Work out the finished part from the listing and answer in its coordinate system (mm). A direction names the side the tool comes from. Coordinates: 2 decimals unless noted, no trailing zeros. Order: outer loops, then holes, each group sorted by start corner. A loop starts at its lowest first (then second) coordinate and runs counter-clockwise, first axis right, second up. Notation, with made-up numbers: M 64,31 L 74,31 A22 ccw 74,63 Z; hole C -20,74.5 d10. An arc over 180 degrees is marked long. Use a Markdown table: item, result.
from build123d import *

# Parameters (mm, degrees)
SKETCH_1_W          = 78
SKETCH_1_H          = 22.5
SKETCH_1_R          = 1
EXTRUDE_1_DEPTH     = 3
FILLET_1_R          = 5
SKETCH_2_R          = 1.5
SKETCH_2_W          = 20
SKETCH_2_H          = 6
EXTRUDE_2_DEPTH     = 3
SKETCH_4_R          = 1.5
CUT_EXTRUDE_1_DEPTH = 29.5
SKETCH_6_R          = 1.5
CUT_EXTRUDE_3_DEPTH = 39
FILLET_7_R          = 6
SKETCH_7_R          = 1.5
CUT_EXTRUDE_4_DEPTH = 10
FILLET_9_R          = 1
FILLET_10_R         = 5


with BuildPart() as part:
    # 草图1 → 凸台-拉伸1 (new body)
    with BuildSketch(Plane(origin=(0, 0, 0), x_dir=(1, 0, 0), z_dir=(0, 1, 0))):
        Rectangle(SKETCH_1_W, SKETCH_1_H)
        with Locations(Location((36, 4, 0), (0, 0, 270))):
            Circle(SKETCH_1_R, mode=Mode.SUBTRACT)
        with Locations(Location((24, 4, 0), (0, 0, 90))):
            Circle(SKETCH_1_R, mode=Mode.SUBTRACT)
        with Locations(Location((36, -4, 0), (0, 0, 90))):
            Circle(SKETCH_1_R, mode=Mode.SUBTRACT)
        with Locations(Location((24, -4, 0), (0, 0, 270))):
            Circle(SKETCH_1_R, mode=Mode.SUBTRACT)
        with Locations(Location((-24, -4, 0), (0, 0, 90))):
            Circle(SKETCH_1_R, mode=Mode.SUBTRACT)
        with Locations(Location((-36, -4, 0), (0, 0, 270))):
            Circle(SKETCH_1_R, mode=Mode.SUBTRACT)
        with Locations(Location((-24, 4, 0), (0, 0, 270))):
            Circle(SKETCH_1_R, mode=Mode.SUBTRACT)
        with Locations(Location((-36, 4, 0), (0, 0, 90))):
            Circle(SKETCH_1_R, mode=Mode.SUBTRACT)
    extrude(amount=EXTRUDE_1_DEPTH)

    # 圆角1
    fillet_1_edges = [part.edges().sort_by_distance(p)[0] for p in [
        (39, 1.5, 11.25),
        (-39, 1.5, 11.25),
        (-39, 1.5, -11.25),
        (39, 1.5, -11.25),
    ]]
    fillet(fillet_1_edges, radius=FILLET_1_R)

    # 草图2 → 凸台-拉伸2 (add)
    # profile 1 of 4: a face of its own
    with BuildSketch(Plane(origin=(0, 3, 0), x_dir=(1, 0, 0), z_dir=(0, 1, 0))):
        Polygon((-10, -31.75), (-10, -11.25), (-18, -11.25), (-18, -37.75), (-10, -37.75), align=None)
        with Locations((-14, -21)):
            Circle(SKETCH_2_R, mode=Mode.SUBTRACT)
    # profile 2 of 4: a face of its own
    with BuildSketch(Plane(origin=(0, 3, 0), x_dir=(1, 0, 0), z_dir=(0, 1, 0))):
        with Locations((-14, -21)):
            Circle(SKETCH_2_R)
    # profile 3 of 4: a face of its own
    with BuildSketch(Plane(origin=(0, 3, 0), x_dir=(1, 0, 0), z_dir=(0, 1, 0))):
        Polygon((18, -11.25), (10, -11.25), (10, -31.75), (10, -37.75), (18, -37.75), align=None)
        with Locations(Location((14, -21, 0), (0, 0, 270))):
            Circle(SKETCH_2_R, mode=Mode.SUBTRACT)
    # profile 4 of 4: a face of its own
    with BuildSketch(Plane(origin=(0, 3, 0), x_dir=(1, 0, 0), z_dir=(0, 1, 0))):
        with Locations((0, -34.75)):
            Rectangle(SKETCH_2_W, SKETCH_2_H)
    extrude(amount=-EXTRUDE_2_DEPTH)

    # 草图4 → 切除-拉伸1 (cut)
    with BuildSketch(Plane(origin=(0, 3, 0), x_dir=(1, 0, 0), z_dir=(0, 1, 0))):
        with Locations(Location((13, 7.25, 0), (0, 0, 270))):
            Circle(SKETCH_4_R)
        with Locations(Location((-13, 7.25, 0), (0, 0, 90))):
            Circle(SKETCH_4_R)
        with Locations(Location((5, 2.25, 0), (0, 0, 270))):
            Circle(SKETCH_4_R)
        with Locations(Location((-5, 2.25, 0), (0, 0, 90))):
            Circle(SKETCH_4_R)
    extrude(amount=-CUT_EXTRUDE_1_DEPTH, mode=Mode.SUBTRACT)

    # 草图6 → 切除-拉伸3 (cut)
    with BuildSketch(Plane(origin=(0, 3, 0), x_dir=(1, 0, 0), z_dir=(0, 1, 0))):
        with Locations(Location((14, -13, 0), (0, 0, 270))):
            Circle(SKETCH_6_R)
    extrude(amount=-CUT_EXTRUDE_3_DEPTH, mode=Mode.SUBTRACT)

    # 圆角7
    fillet_7_edges = [part.edges().sort_by_distance(p)[0] for p in [
        (-18, 1.5, 11.25),
        (18, 1.5, 11.25),
    ]]
    fillet(fillet_7_edges, radius=FILLET_7_R)

    # 草图7 → 切除-拉伸4 (cut)
    with BuildSketch(Plane(origin=(0, 3, 0), x_dir=(1, 0, 0), z_dir=(0, 1, 0))):
        with Locations(Location((14, -34, 0), (0, 0, 270))):
            Circle(SKETCH_7_R)
        with Locations(Location((-14, -34, 0), (0, 0, 90))):
            Circle(SKETCH_7_R)
    extrude(amount=-CUT_EXTRUDE_4_DEPTH, mode=Mode.SUBTRACT)

    # 圆角9
    fillet_9_edges = [part.edges().sort_by_distance(p)[0] for p in [
        (18, 1.5, 37.75),
        (-18, 1.5, 37.75),
    ]]
    fillet(fillet_9_edges, radius=FILLET_9_R)

    # 圆角10
    fillet_10_edges = [part.edges().sort_by_distance(p)[0] for p in [
        (-10, 1.5, 11.25),
        (-10, 1.5, 31.75),
        (10, 1.5, 31.75),
        (10, 1.5, 11.25),
    ]]
    fillet(fillet_10_edges, radius=FILLET_10_R)


solid = part.part
1. Find the intervals of material crossed by probe 1 along X at (y, z) = (2, -4); probe 2 along X at (y, z) = (1.05, 21); probe 3 along X at (y, z) = (1, -2.25), in increasing order.
Answers below:
| item | result |
|---|---|
| probe 1 | -39 to -37, -35 to -25, -23 to 23, 25 to 35, 37 to 39 |
| probe 2 | -18 to -10, 10 to 12.5, 15.5 to 18 |
| probe 3 | -39 to -6.5, -3.5 to 3.5, 6.5 to 39 |
2. Section D-D on y = 1.35 is taken. Give the number of separate pieces and of enclosed holes in the cut face, then the cut area to 3 significant figures.
Answers below:
| item | result |
|---|---|
| separate pieces | 1 |
| enclosed holes | 17 |
| area | 2,230 mm² |
3. Section A-A on z = 34 is taken. Determine the outline of the cut face in (x, y), then the cut area to 3 significant figures.
Answers below:
| item | result |
|---|---|
| outline | M -18,0 L -15.5,0 L -15.5,3 L -18,3 Z; M -12.5,0 L 12.5,0 L 12.5,3 L -12.5,3 Z; M 15.5,0 L 18,0 L 18,3 L 15.5,3 Z |
| area | 90.0 mm² |
4. For faces 1 (the face through (18, 2, 27)), 2 (the face through (8.5, 1.48, 12.68)), 3 (the face through (-1, 3, 7)), 4 (the face through (-18, 2, 27)), determine the directions among +Z, -Z, +X, -X, +Y, -Y from which every point of the face is accessible in a straight line to the end or side of a thin tool.
Answers below:
| item | result |
|---|---|
| face 1 | +Z, +X, +Y, -Y |
| face 2 | +Y, -Y |
| face 3 | +Z, -Z, +X, -X, +Y |
| face 4 | +Z, -X, +Y, -Y |
5. For a pull along X with two mould halves and no side action, classify faces 5 (the face through (0, 1, -11.25)), 6 (the face through (-13.1, 1.5, 35.2)), 7 (the face through (25, 1, -4)), 8 (the face through (39, 1, 0)) as +X half, -X half, draft (parallel to the pull), parting line (faces both ways), or undercut.
Answers below:
| item | result |
|---|---|
| face 5 | draft |
| face 6 | undercut |
| face 7 | undercut |
| face 8 | +X half |
6. Section B-B on z = 15.5 is taken. Determine the outline of the cut face in (x, y), then the cut area to 3 significant figures.
Answers below:
| item | result |
|---|---|
| outline | M -18.26,0 L -9.94,0 L -9.94,3 L -18.26,3 Z; M 9.94,0 L 18.26,0 L 18.26,3 L 9.94,3 Z |
| area | 49.9 mm² |
7. Flat-ended cylindrical pins translate along their axes: P1, Ø2, axis at x = -6.5, z = 14, coming from the +Y side; P2, Ø3, axis at x = 24, z = 4, coming from the +Y side; P3, Ø0.9, axis at y = 2, z = 19.5, coming from the +X side; P4, Ø1, axis at y = 2.5, z = 18, coming from the -X side. Find the tip coordinate at first contact, or state that the pin passes through.
Answers below:
| item | result |
|---|---|
| P1 | through |
| P2 | y = 3 |
| P3 | x = 18 |
| P4 | x = -18 |
8. Section C-C on x = -36 is taken. Determine the outline of the cut face in (y, z).
Answers below:
| item | result |
|---|---|
| outline | M 0,-10.83 L 3,-10.83 L 3,-5 L 0,-5 Z; M 0,-3 L 3,-3 L 3,3 L 0,3 Z; M 0,5 L 3,5 L 3,10.83 L 0,10.83 Z |
